Work out the finished part from the listing and answer in its coordinate system (mm). A direction names the side the tool comes from. Round coordinates to 2 decimals unless told otherwise and drop trailing zeros. Write each loop counter-clockwise with the first axis right and the second up, starting at its lowest first coordinate (ties: lowest second). Pieces come first, ordered by that corner, then holes. Notation, with made-up numbers: (-27.75, 9.25) - (-13.75, 9.25) arc R12 ccw to (-13.75, 31.25) - close; hole circle Ø7 at (56, 45.5). An arc over 180 degrees is marked (long way). Write item = value, one per line. Start each with the question number.
Autodesk Inventor part; units mm, degrees
ref_plane "YZ Plane" through (0, 0, 0) normal (1, 0, 0) x (0, 1, 0)
ref_plane "XZ Plane" through (0, 0, 0) normal (0, 1, 0) x (-1, 0, 0)
ref_plane "XY Plane" through (0, 0, 0) normal (0, 0, 1) x (1, 0, 0)
sketch "Sketch1" plane through (0, 0, 0) normal (0, 1, 0) x (-1, 0, 0)
  line L0 (15.24, -15.24) -> (-15.24, -15.24)
  line L1 (-15.24, -15.24) -> (-15.24, 15.24)
  line L2 (-15.24, 15.24) -> (15.24, 15.24)
  line L3 (15.24, 15.24) -> (15.24, -15.24)
  line L4 (15.24, -15.24) -> (-15.24, 15.24) construction
  line L5 (-15.24, -15.24) -> (15.24, 15.24) construction
  circle A0 centre (0, 0) radius 15.24
  dimension "d0" = 30.48
  dimension "d3" = 30.48
extrude "Extrusion1" add sketch "Sketch1" along normal blind 2.54
sketch "Sketch2" plane through (-15.24, 0, 15.24) normal (0, 0, 1) x (1, 0, 0)
  line L0 (30.48, 0) -> (0, 0)
  line L1 (8.8466, 2.54) -> (21.6334, 2.54)
  line L2 (21.6334, 2.54) -> (21.6334, 0)
  line L3 (21.6334, 0) -> (8.8466, 0)
  line L4 (8.8466, 0) -> (8.8466, 2.54)
  line L5 (8.8466, 2.54) -> (21.6334, 0) construction
  line L6 (21.6334, 2.54) -> (8.8466, 0) construction
  point P0 (15.24, 0)
  point P1 (15.24, 1.27)
extrude "Extrusion2" add sketch "Sketch2" along normal blind 63.5
sketch "Sketch5" plane through (-15.24, 0, 78.74) normal (0, 0, 1) x (1, 0, 0)
  circle A0 centre (15.24, 1.27) radius 6.35
  point P0 (15.24, 0)
  dimension "d14" = 12.7
extrude "Extrusion5" add sketch "Sketch5" along normal blind 25.4
sketch "Sketch7" plane through (15.24, 0, 15.24) normal (1, 0, 0) x (0, 0, -1)
  line L0 (1.27, 2.032) -> (29.21, 2.032)
  line L1 (29.21, 2.032) -> (29.21, 0.508)
  line L2 (29.21, 0.508) -> (1.27, 0.508)
  line L3 (1.27, 0.508) -> (1.27, 2.032)
  line L4 (1.27, 2.032) -> (29.21, 0.508) construction
  line L5 (29.21, 2.032) -> (1.27, 0.508) construction
  point P0 (15.24, 0)
  point P1 (15.24, 1.27)
  dimension "d35" = 27.94
  dimension "d36" = 1.524
extrude "Extrusion7" cut sketch "Sketch7" against normal blind 15.24
sketch "Sketch8" plane through (0, 2.54, 0) normal (0, 1, 0) x (1, 0, 0)
  circle A0 centre (0, 0) radius 12.065
  dimension "d39" = 24.13
extrude "Extrusion8" cut sketch "Sketch8" against normal blind 31.75
sketch "Sketch9" plane through (0, 2.54, 0) normal (0, 1, 0) x (1, 0, 0)
  circle A0 centre (0, 0) radius 12.065
  line L0 (15.24, 15.24) -> (-15.24, 15.24)
  line L1 (-15.24, 15.24) -> (-15.24, -15.24)
  line L2 (-15.24, -15.24) -> (-6.3934, -15.24)
  line L3 (-6.3934, -15.24) -> (-6.3934, -78.74)
  line L4 (-6.2217, -78.74) -> (-6.3934, -78.74)
  line L5 (6.2217, -78.74) -> (-6.2217, -78.74)
  line L6 (6.3934, -78.74) -> (6.2217, -78.74)
  line L7 (6.3934, -15.24) -> (6.3934, -78.74)
  line L8 (6.3934, -15.24) -> (15.24, -15.24)
  line L9 (15.24, -15.24) -> (15.24, 15.24)
  circle A1 centre (0, 0) radius 13.97
  circle A2 centre (0, 0) radius 12.065
  line L10 (-6.2217, -78.74) -> (6.2217, -78.74)
  line L11 (6.2217, -78.74) -> (6.2217, -104.14)
  line L12 (6.2217, -104.14) -> (-6.2217, -104.14)
  line L13 (-6.2217, -104.14) -> (-6.2217, -78.74)
  line L14 (-6.2217, -78.74) -> (-6.3934, -78.74)
  line L15 (-6.3934, -78.74) -> (-6.3934, -15.24)
  line L16 (-6.3934, -15.24) -> (-15.24, -15.24)
  line L17 (-15.24, -15.24) -> (-15.24, 15.24)
  line L18 (-15.24, 15.24) -> (15.24, 15.24)
  line L19 (15.24, 15.24) -> (15.24, -15.24)
  line L20 (15.24, -15.24) -> (6.3934, -15.24)
  line L21 (6.3934, -15.24) -> (6.3934, -78.74)
  line L22 (6.3934, -78.74) -> (6.2217, -78.74)
  dimension "d42" = 27.94
properties part number "Silicon Frame v2"
1. Which of the six approach directions +Z, -Z, +X, -X, +Y, -Y give full straight-line access (tool end or side, diameter ignored) to faces 4 (the face through (0, 0, 32)), 5 (the face through (6.393, 1, 47)), 6 (the face through (0, 5, 78.74)), 7 (the face through (13, 2.032, 0))?
2. Consider line 1 (Z direction, x = 0, y = 2.5) (3 decimals); line 2 (Y direction, x = 10, z = 14); line 3 (Z direction, x = -3, y = -3). Determine where each line is inside the solid, lowest interval first.
3. Find section C-C on x = -9.5. Give the vertices of the cut face in (y, z), plus the area to 3 significant figures.
4. Find section A-A on z = 0. Give the vertices of the cut face in (x, y) (3 decimals).
5. Find section D-D on z = 39.5. Give the vertices of the cut face in (x, y), plus the area to 3 significant figures.
6. Each of these flat-tipped pins is pushed along its axis until it touches: pin 1 (4.5 mm diameter, centred on x = 7.5, z = 1.5, fed in from -Y); pin 2 (15 mm diameter, centred on x = -1.5, z = 36.5, fed in from +Y); pin 3 (0.8 mm diameter, centred on y = 1, z = 13, fed in from +X); pin 4 (3 mm diameter, centred on x = 9, y = 1, fed in from +Z). Where does it stop, or does it pass through?
7. For a pull along Y with two mould halves and no side action, classify faces 1 (the face through (13, 0.508, 0)), 2 (the face through (-6.393, 1, 47)), 3 (the face through (0, 2.54, 32)) as released by +Y, released by -Y, zero draft, split by the parting line, or undercut.
8. Find section B-B on x = 8.5. Give the vertices of the cut face in (y, z).
Answer key:
q1.face_4 = -Z, +X, -X, -Y
q1.face_5 = +Z, +X, +Y, -Y
q1.face_6 = -Z, +X, -X, +Y
q1.face_7 = +X
q2.line_1 = -15.24 to -12.065, 12.065 to 104.14
q2.line_2 = 0 to 2.54
q2.line_3 = 78.74 to 104.14
q3.outline = (0, -15.24) - (2.54, -15.24) - (2.54, -7.44) - (0, -7.44) - close; (0, 7.44) - (2.54, 7.44) - (2.54, 15.24) - (0, 15.24) - close
q3.area = 39.6 mm²
q4.outline = (-15.24, 0) - (-12.065, 0) - (-12.065, 2.54) - (-15.24, 2.54) - close; (12.065, 0) - (15.24, 0) - (15.24, 0.508) - (12.065, 0.508) - close; (12.065, 2.032) - (15.24, 2.032) - (15.24, 2.54) - (12.065, 2.54) - close
q5.outline = (-6.39, 0) - (6.39, 0) - (6.39, 2.54) - (-6.39, 2.54) - close
q5.area = 32.5 mm²
q6.pin_1 = through
q6.pin_2 = 2.54
q6.pin_3 = 0
q6.pin_4 = 15.24
q7.face_1 = undercut
q7.face_2 = zero draft
q7.face_3 = released by +Y
q8.outline = (0, -15.24) - (2.54, -15.24) - (2.54, -8.56) - (2.03, -8.56) - (2.03, -13.97) - (0.51, -13.97) - (0.51, -8.56) - (0, -8.56) - close; (0, 8.56) - (0.51, 8.56) - (0.51, 13.97) - (2.03, 13.97) - (2.03, 8.56) - (2.54, 8.56) - (2.54, 15.24) - (0, 15.24) - close
